Can you work these out from the model? Positions are in its coordinate system, mm. A direction names the side the tool comes from. Coordinates: 2 decimals unless noted, no trailing zeros. Write each loop counter-clockwise with the first axis right and the second up, starting at its lowest first coordinate (ties: lowest second). Pieces come first, ordered by that corner, then holes. Notation, with made-up numbers: (47, 55) -> (72, 55) arc R20 ccw to (72, 89) -> close; hole circle Ø11 at (34, 42). An arc over 180 degrees is marked (long way). Answer as CSV lines item,"result". Start each with the question number.
```python
from build123d import *

# Parameters (mm, degrees)
BOSS_EXTRU_1_DEPTH      = 10
ESQUISSE2_R             = 1.025
ENL_V_MAT_EXTRU_1_DEPTH = 8
ENL_V_MAT_EXTRU_2_REACH = 130.997
ESQUISSE3_R             = 1.75
ESQUISSE4_R             = 3.5
ESQUISSE4_R_2           = 1.75
ENL_V_MAT_EXTRU_3_DEPTH = 4
BOSS_EXTRU_2_DEPTH      = 10
ESQUISSE6_R             = 2.75
ENL_V_MAT_EXTRU_4_DEPTH = 2


with BuildPart() as part:
    # Esquisse1 → Boss.-Extru.1 (new body)
    with BuildSketch(Plane.XY):
        with BuildLine():
            Line((-12.5, -128), (12.5, -128))
            Line((12.5, -128), (10.205358779, -104.502873894))
            ThreePointArc((10.205358779, -104.502873894), (0, -105), (-10.205358779, -104.502873894))
            Line((-10.205358779, -104.502873894), (-12.5, -128))
        make_face()
    extrude(amount=BOSS_EXTRU_1_DEPTH)

    # Esquisse2 → Enlèv. mat.-Extru.1 (cut)
    with BuildSketch(Plane.XZ.offset(128)):
        with Locations((-4.75, 6)):
            Circle(ESQUISSE2_R)
        with Locations((4.75, 6)):
            Circle(ESQUISSE2_R)
    extrude(amount=-ENL_V_MAT_EXTRU_1_DEPTH, mode=Mode.SUBTRACT)

    # Esquisse3 → Enlèv. mat.-Extru.2 (cut, up to next)
    with BuildSketch(Plane.XY.offset(10), mode=Mode.PRIVATE) as enl_v_mat_extru_2_sk1:
        with Locations((-7.020582047, -114.785501819)):
            Circle(ESQUISSE3_R)
    enl_v_mat_extru_2_tool1 = extrude(enl_v_mat_extru_2_sk1.sketch, amount=-ENL_V_MAT_EXTRU_2_REACH, mode=Mode.PRIVATE) & part.part
    # Esquisse3 → Enlèv. mat.-Extru.2 (cut, up to next)
    with BuildSketch(Plane.XY.offset(10), mode=Mode.PRIVATE) as enl_v_mat_extru_2_sk2:
        with Locations((7.020582047, -114.785501819)):
            Circle(ESQUISSE3_R)
    enl_v_mat_extru_2_tool2 = extrude(enl_v_mat_extru_2_sk2.sketch, amount=-ENL_V_MAT_EXTRU_2_REACH, mode=Mode.PRIVATE) & part.part
    add(enl_v_mat_extru_2_tool1.solids().sort_by_distance((-7.020582, -114.785502, 10))[0], mode=Mode.SUBTRACT)
    add(enl_v_mat_extru_2_tool2.solids().sort_by_distance((7.020582, -114.785502, 10))[0], mode=Mode.SUBTRACT)

    # Esquisse4 → Enlèv. mat.-Extru.3 (cut)
    # profile 1 of 2: a face of its own
    with BuildSketch(Plane.XY.offset(10)):
        with Locations((7.020582047, -114.785501819)):
            Circle(ESQUISSE4_R)
        with Locations((7.020582047, -114.785501819)):
            Circle(ESQUISSE4_R_2, mode=Mode.SUBTRACT)
    # profile 2 of 2: a face of its own
    with BuildSketch(Plane.XY.offset(10)):
        with Locations((-7.020582047, -114.785501819)):
            Circle(ESQUISSE4_R)
    extrude(amount=-ENL_V_MAT_EXTRU_3_DEPTH, mode=Mode.SUBTRACT)

    # Esquisse5 → Boss.-Extru.2 (add)
    with BuildSketch(Plane.XY.offset(10)):
        Polygon((-12.5, -140.725580344), (-21.915902578, -139.56945288), (-10.205358779, -104.502873894), (-12.5, -128), align=None)
    extrude(amount=-BOSS_EXTRU_2_DEPTH)

    # Esquisse6 → Enlèv. mat.-Extru.4 (cut)
    with BuildSketch(Plane(origin=(-17.207951289, -140.147516612, 0), x_dir=(0.9925461516413231, -0.12186934340513994, 0), z_dir=(-0.12186934340513994, -0.9925461516413231, 0))):
        with Locations((0, 5)):
            Circle(ESQUISSE6_R)
    extrude(amount=-ENL_V_MAT_EXTRU_4_DEPTH, mode=Mode.SUBTRACT)


solid = part.part
```
Q1. Imagine slicing it at B-B (x = 6.5). Write out the boundary of the cut face in (y, z).
Q2. For pin 1 (3 mm diameter, centred on x = -7.02, y = -114.79, fed in from -Z); pin 2 (1.6 mm diameter, centred on x = -4.75, z = 6, fed in from -Y); pin 3 (1 mm diameter, centred on y = -134.5, z = 7.5, fed in from +X); pin 4 (1 mm diameter, centred on x = -5, z = 6.5, fed in from -Y), each with a flat end and sliding along its axis, tell me the tip position at first contact or that it passes through.
Q3. Imagine slicing it at C-C (z = 6.5). Write out the boundary of the cut face in (x, y).
Q4. Imagine slicing it at A-A (y = -115.5). Write out the boundary of the cut face in (x, z), then the cut area to 3 significant figures.
Q5. Imagine slicing it at D-D (z = 2.75). Write out the boundary of the cut face in (x, y), then the cut area to 3 significant figures.
Q6. Which directions (+Z, -Z, +X, -X, +Y, -Y) give clear straight access to the entire face, cutting with the end or side of a thin tool? Please do faces 1 (the face through (-4, -118, 0)), 2 (the face through (-19.254, -138.903, 3.327)), 3 (the face through (5, -120, 6)), 4 (the face through (-9, -116, 6)), 5 (the face through (-12.5, -134, 5)).
Q7. I need wall thicknesses on L1, parallel to X at y = -115.5, z = 6.25; L2, parallel to X at y = -115, z = 3.75; L3, parallel to Y at x = -4.5, z = 8.5. Which ranges of each line are inside material? Lowest first, please.
Q8. If we mould it in two halves opening along X, with no side actions, what happens to faces 6 (the face through (-7.779, -118.202, 8.028)), 7 (the face through (11.37, -116.42, 4.93)), 8 (the face through (0, -128, 5))? For each: released by +X, released by -X, zero draft, split by the parting line, or undercut.
Entries:
1,outline,"(-128, 0) -> (-116.46, 0) -> (-116.46, 6) -> (-118.25, 6) -> (-118.25, 10) -> (-128, 10) -> close; (-113.11, 0) -> (-104.8, 0) -> (-104.8, 10) -> (-111.32, 10) -> (-111.32, 6) -> (-113.11, 6) -> close"
2,pin 1,"through"
2,pin 2,"y = -120"
2,pin 3,"x = -12.5"
2,pin 4,"y = -128"
3,outline,"(-21.92, -139.57) -> (-19.5, -139.87) -> (-19.25, -137.88) -> (-14.68, -138.44) -> (-14.92, -140.43) -> (-12.5, -140.73) -> (-12.5, -128) -> (-5.64, -128) -> (-5.64, -120) -> (-3.86, -120) -> (-3.86, -128) -> (3.86, -128) -> (3.86, -120) -> (5.64, -120) -> (5.64, -128) -> (12.5, -128) -> (10.21, -104.5) arc R105 cw to (-10.21, -104.5) -> close; hole circle Ø7 at (-7.02, -114.79); hole circle Ø7 at (7.02, -114.79)"
4,outline,"(-13.88, 0) -> (-8.62, 0) -> (-8.62, 6) -> (-10.45, 6) -> (-10.45, 10) -> (-13.88, 10) -> close; (-5.42, 0) -> (5.42, 0) -> (5.42, 6) -> (3.59, 6) -> (3.59, 10) -> (-3.59, 10) -> (-3.59, 6) -> (-5.42, 6) -> close; (8.62, 0) -> (11.28, 0) -> (11.28, 10) -> (10.45, 10) -> (10.45, 6) -> (8.62, 6) -> close"
4,area,"158 mm2"
5,outline,"(-21.92, -139.57) -> (-18.78, -139.95) -> (-18.53, -137.97) -> (-15.39, -138.36) -> (-15.64, -140.34) -> (-12.5, -140.73) -> (-12.5, -128) -> (12.5, -128) -> (10.21, -104.5) arc R105 cw to (-10.21, -104.5) -> close; hole circle Ø3.5 at (-7.02, -114.79); hole circle Ø3.5 at (7.02, -114.79)"
5,area,"658 mm2"
6,face 1,"-Z, +X, -X, +Y, -Y"
6,face 2,"none"
6,face 3,"-Y"
6,face 4,"+Z"
6,face 5,"+Z, -Z, +X, -Y"
7,L1,"-13.88 to -10.45, -3.59 to 3.59, 10.45 to 11.28"
7,L2,"-13.71 to -8.76, -5.28 to 5.28, 8.76 to 11.23"
7,L3,"-128 to -117.21, -112.36 to -104.9"
8,face 6,"undercut"
8,face 7,"released by +X"
8,face 8,"zero draft"
